Work out the finished part from the listing and answer in its coordinate system (mm). A direction names the side the tool comes from. Round coordinates to 2 decimals unless told otherwise and drop trailing zeros. Order: outer loops, then holes, each group sorted by start corner. A loop starts at its lowest first (then second) coordinate and runs counter-clockwise, first axis right, second up. Notation, with made-up numbers: (35, 87.25) - (59, 87.25) arc R25 cw to (59, 124.25) - close; hole circle Ø4 at (68, 37). An arc over 180 degrees is marked (long way). Use one line per item in the form item = value. Start each with the question number.
Q1. Which of the six approach directions +Z, -Z, +X, -X, +Y, -Y give full straight-line access (tool end or side, diameter ignored) to faces 4 (the cylindrical face through (30.497, 3.972, -0.286)), 5 (the flat face through (0, 4, 13)), 6 (the cylindrical face through (-29.497, 3.261, -0.264))?
Q2. The part is cut by section A-A on y = 12.75. Determine the outline of the cut face in (x, z), plus the area to 3 significant figures.
Q3. For a pull along X with two mould halves and no side action, classify faces 1 (the cylindrical face through (-2.777, 13.958, 6.697)), 2 (the flat face through (0, 9, -10)), 3 (the cylindrical face through (-31.61, 0.49, 11.56)) as +X half, -X half, draft (parallel to the pull), parting line (faces both ways), or undercut.
Q4. Find the intervals of material crossed by line 1 (X direction, y = 0.9, z = -13); line 2 (X direction, y = 1.5, z = -13); line 3 (Z direction, x = -9, y = 5.5), in increasing order. Write a range as [from, to].
Q5. Given P1, Ø4.5, axis at x = -9.5, z = -0.5, coming from the -Y side; P2, Ø3, axis at x = -18.5, z = 11.5, coming from the +Y side; P3, Ø3, axis at x = -33, z = -13, coming from the +Y side, each flat-ended and moving along its own axis, determine where each tip first touches the part or whether it passes through.
from build123d import *

# Parameters (mm, degrees)
SKETCH_1_W          = 70
SKETCH_1_H          = 30
EXTRUDE_1_DEPTH     = 2
SKETCH_2_R          = 1
CUT_EXTRUDE_1_DEPTH = 39.13135193
EXTRUDE_2_DEPTH     = 9
CHAMFER_2_SIZE      = 5
SHELL_2_DEPTH       = 5.585786438
SHELL_2_2_DEPTH     = 1
SKETCH_4_R          = 7.25
EXTRUDE_3_DEPTH     = 6


with BuildPart() as part:
    # 草图1 → 凸台-拉伸1 (new body)
    with BuildSketch(Plane(origin=(0, 0, 0), x_dir=(1, 0, 0), z_dir=(0, 1, 0))):
        Rectangle(SKETCH_1_W, SKETCH_1_H)
    extrude(amount=EXTRUDE_1_DEPTH)

    # 草图2 → 切除-拉伸1 (cut, through all)
    with BuildSketch(Plane(origin=(0, 2, 0), x_dir=(1, 0, 0), z_dir=(0, 1, 0))):
        with Locations(Location((-33, 13, 0), (0, 0, 270))):
            Circle(SKETCH_2_R)
        with Locations(Location((33, 13, 0), (0, 0, 90))):
            Circle(SKETCH_2_R)
        with Locations(Location((33, -13, 0), (0, 0, 270))):
            Circle(SKETCH_2_R)
        with Locations(Location((-33, -13, 0), (0, 0, 90))):
            Circle(SKETCH_2_R)
    extrude(amount=-CUT_EXTRUDE_1_DEPTH, mode=Mode.SUBTRACT)

    # 草图3 → 凸台-拉伸2 (add)
    with BuildSketch(Plane(origin=(0, 2, 0), x_dir=(1, 0, 0), z_dir=(0, 1, 0))):
        with BuildLine():
            Line((-17.5, 13), (17.5, 13))
            ThreePointArc((17.5, 13), (30.5, 0), (17.5, -13))
            Line((17.5, -13), (-17.5, -13))
            ThreePointArc((-17.5, -13), (-30.5, 0), (-17.5, 13))
        make_face()
    extrude(amount=EXTRUDE_2_DEPTH)

    # 倒角2
    chamfer_2_edges = [part.edges().sort_by_distance(p)[0] for p in [
        (-30.5, 11, 0),
        (0, 11, 13),
        (30.5, 11, 0),
        (0, 11, -13),
    ]]
    chamfer(chamfer_2_edges, length=CHAMFER_2_SIZE)

    # 抽壳2: read off the stored shape, not the designer's step
    # 抽壳2 outline → 抽壳2 (cut)
    with BuildSketch(Plane(origin=(0, 0, 0), x_dir=(1, 0, 0), z_dir=(0, 1, 0))):
        with BuildLine():
            ThreePointArc((-17.5, 12), (-29.5, 0), (-17.5, -12))
            Line((-17.5, -12), (17.5, -12))
            ThreePointArc((17.5, -12), (29.5, 0), (17.5, 12))
            Line((17.5, 12), (-17.5, 12))
        make_face()
    extrude(amount=SHELL_2_DEPTH, mode=Mode.SUBTRACT)

    # Shell 2 2 outline → Shell 2 2 (cut)
    with BuildSketch(Plane(origin=(0, 0, 0), x_dir=(1, 0, 0), z_dir=(0, 1, 0))):
        with BuildLine():
            Line((-34, 11.267949192), (-34, -11.267949192))
            ThreePointArc((-34, -11.267949192), (-31.585786438, -11.585786438), (-31.267949192, -14))
            Line((-31.267949192, -14), (31.267949192, -14))
            ThreePointArc((31.267949192, -14), (31.585786438, -11.585786438), (34, -11.267949192))
            Line((34, -11.267949192), (34, 11.267949192))
            ThreePointArc((34, 11.267949192), (31.585786438, 11.585786438), (31.267949192, 14))
            Line((31.267949192, 14), (-31.267949192, 14))
            ThreePointArc((-31.267949192, 14), (-31.585786438, 11.585786438), (-34, 11.267949192))
        make_face()
        with BuildLine():
            Line((17.5, -12), (-17.5, -12))
            ThreePointArc((-17.5, -12), (-29.5, 0), (-17.5, 12))
            Line((-17.5, 12), (17.5, 12))
            ThreePointArc((17.5, 12), (29.5, 0), (17.5, -12))
        make_face(mode=Mode.SUBTRACT)
    extrude(amount=SHELL_2_2_DEPTH, mode=Mode.SUBTRACT)

    # Shell 2 3: loft between two sections, ruled curve by curve
    shell_2_3_from = [
        Edge.make_three_point_arc((17.5, 10, -7.585786438), (22.863961031, 10, -5.363961031), (25.085786438, 10, 0)),
        Edge.make_three_point_arc((25.085786438, 10, 0), (22.863961031, 10, 5.363961031), (17.5, 10, 7.585786438)),
        Edge.make_three_point_arc((-17.5, 10, 7.585786438), (-22.863961031, 10, 5.363961031), (-25.085786438, 10, 0)),
        Edge.make_three_point_arc((-25.085786438, 10, 0), (-22.863961031, 10, -5.363961031), (-17.5, 10, -7.585786438)),
        Edge.make_line((17.5, 10, -7.585786438), (-17.5, 10, -7.585786438)),
        Edge.make_line((17.5, 10, 7.585786438), (-17.5, 10, 7.585786438)),
    ]
    shell_2_3_to = [
        Edge.make_three_point_arc((17.5, 5.585786438, -12), (25.985281374, 5.585786438, -8.485281374), (29.5, 5.585786438, 0)),
        Edge.make_three_point_arc((29.5, 5.585786438, 0), (25.985281374, 5.585786438, 8.485281374), (17.5, 5.585786438, 12)),
        Edge.make_three_point_arc((-17.5, 5.585786438, 12), (-25.985281374, 5.585786438, 8.485281374), (-29.5, 5.585786438, 0)),
        Edge.make_three_point_arc((-29.5, 5.585786438, 0), (-25.985281374, 5.585786438, -8.485281374), (-17.5, 5.585786438, -12)),
        Edge.make_line((17.5, 5.585786438, -12), (-17.5, 5.585786438, -12)),
        Edge.make_line((17.5, 5.585786438, 12), (-17.5, 5.585786438, 12)),
    ]
    shell_2_3 = Solid(Shell([*[Face.make_surface_from_curves(shell_2_3_from[k], shell_2_3_to[k]) for k in range(6)], Face(Wire(shell_2_3_from)), Face(Wire(shell_2_3_to))]))
    add(shell_2_3, mode=Mode.SUBTRACT)

    # 草图4 → 凸台-拉伸3 (add)
    with BuildSketch(Plane(origin=(0, 11, 0), x_dir=(1, 0, 0), z_dir=(0, 1, 0))):
        with Locations(Location((0, 0, 0), (0, 0, 270))):
            Circle(SKETCH_4_R)
    extrude(amount=EXTRUDE_3_DEPTH)


solid = part.part
Found:
q1.face_4 = +X, +Y
q1.face_5 = +Z, +X, -X, +Y
q1.face_6 = -Y
q2.outline = circle Ø14.5 at (0, 0)
q2.area = 165 mm²
q3.face_1 = parting line
q3.face_2 = draft
q3.face_3 = undercut
q4.line_1 = [-35, -34], [-32, -31], [31, 32], [34, 35]
q4.line_2 = [-35, -34], [-32, 32], [34, 35]
q4.line_3 = [-13, -12], [12, 13]
q5.P1 = 10
q5.P2 = 8.96
q5.P3 = 2
